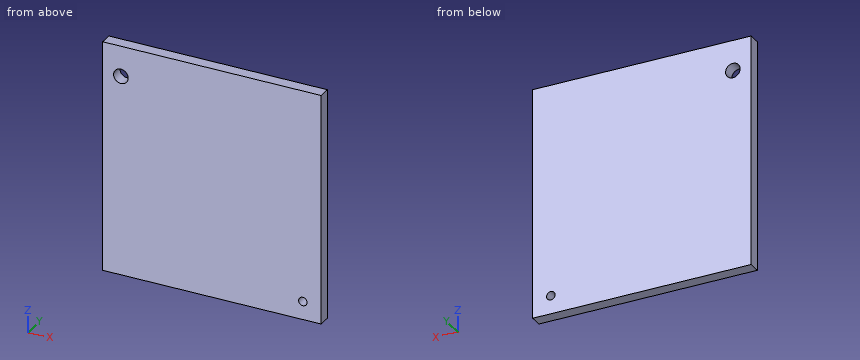
```python
from build123d import *

# Parameters (mm, degrees)
SKETCH1_W           = 180
SKETCH1_H           = 190
BOSS_EXTRUDE1_DEPTH = 10
SKETCH2_R           = 3.5
CUT_EXTRUDE1_DEPTH  = 11
SKETCH6_R           = 6
CUT_EXTRUDE2_DEPTH  = 11


with BuildPart() as part:
    # Sketch1 → Boss-Extrude1 (new body)
    with BuildSketch(Plane(origin=(0, 0, 0), x_dir=(1, 0, 0), z_dir=(0, 1, 0))):
        with Locations((0, -5)):
            Rectangle(SKETCH1_W, SKETCH1_H)
    extrude(amount=BOSS_EXTRUDE1_DEPTH)

    # Sketch2 → Cut-Extrude1 (cut, through all)
    with BuildSketch(Plane(origin=(0, 10, 0), x_dir=(1, 0, 0), z_dir=(0, 1, 0))):
        with Locations((75, 75)):
            Circle(SKETCH2_R)
    extrude(amount=-CUT_EXTRUDE1_DEPTH, mode=Mode.SUBTRACT)

    # Sketch6 → Cut-Extrude2 (cut, through all)
    with BuildSketch(Plane(origin=(0, 10, 0), x_dir=(1, 0, 0), z_dir=(0, 1, 0))):
        with Locations((-75, -75)):
            Circle(SKETCH6_R)
    extrude(amount=-CUT_EXTRUDE2_DEPTH, mode=Mode.SUBTRACT)


solid = part.part
```
Check sheet for the modelled part. Datum: model origin and axes. Units: mm. Give positions to 0.01 mm unless a question says otherwise; leave off trailing zeros. Loops run counter-clockwise (first coordinate to the right, second up) from the corner with the lowest first, then second, coordinate; pieces in that order, holes last. Notation, with made-up numbers: M 3.25,86 L 32.25,86 A11 ccw 32.25,94 Z; hole C -1,64 d8. An arc over 180 degrees is marked long. Answer in a Markdown table with one row per item.
1) Thickness scan on line 1 (Z direction, x = -75, y = 3.25); line 2 (X direction, y = 7.5, z = -75); line 3 (X direction, y = 8.25, z = 75). Record the ranges inside material, lowest first.
Solutions:
| item | result |
|---|---|
| line 1 | z = -90 to 69, 81 to 100 |
| line 2 | x = -90 to 71.5, 78.5 to 90 |
| line 3 | x = -90 to -81, -69 to 90 |
2) Depth check by flat-ended pin: pin 1 (6.5 mm diameter, centred on x = 75, z = -75, fed in from +Y). Enter the tip coordinate at first touch or a pass-through.
Solutions:
| item | result |
|---|---|
| pin 1 | passes through |
3) Cross-section at B-B (z = 75). Enter the section's corners in (x, y).
Solutions:
| item | result |
|---|---|
| outline | M -90,0 L -81,0 L -81,10 L -90,10 Z; M -69,0 L 90,0 L 90,10 L -69,10 Z |
4) Cross-section at A-A (x = -75). Enter the section's corners in (y, z), plus the area to 3 significant figures.
Solutions:
| item | result |
|---|---|
| outline | M 0,-90 L 10,-90 L 10,69 L 0,69 Z; M 0,81 L 10,81 L 10,100 L 0,100 Z |
| area | 1,780 mm^2 |
